Design review of the part built by this model. Coordinates are the model's own, in mm. A direction names the side the tool comes from. Coordinates: 2 decimals unless noted, no trailing zeros. Loops run counter-clockwise (first coordinate to the right, second up) from the corner with the lowest first, then second, coordinate; pieces in that order, holes last. Notation, with made-up numbers: (10.25, 12) -> (49.25, 12) arc R7 ccw to (49.25, 19) -> close; hole circle Ø10 at (45.25, 45). An arc over 180 degrees is marked (long way). Answer as a JSON object with one key per item and string values.
Autodesk Inventor part; units mm, degrees
ref_plane "YZ Plane" through (0, 0, 0) normal (1, 0, 0) x (0, 1, 0)
ref_plane "XZ Plane" through (0, 0, 0) normal (0, 1, 0) x (-1, 0, 0)
ref_plane "XY Plane" through (0, 0, 0) normal (0, 0, 1) x (1, 0, 0)
sketch "Sketch - Main Body" plane through (0, 0, 0) normal (0, 1, 0) x (-1, 0, 0)
  line L0 (-16.925, 11.65) -> (16.925, 11.65)
  line L1 (16.925, 11.65) -> (16.925, -11.65)
  line L2 (16.925, -11.65) -> (-16.925, -11.65)
  line L3 (-16.925, -11.65) -> (-16.925, 11.65)
  line L4 (-16.925, 11.65) -> (16.925, -11.65) construction
  line L5 (16.925, 11.65) -> (-16.925, -11.65) construction
  line L6 (-16.65, 11.25) -> (16.65, 11.25)
  line L7 (16.65, -11.25) -> (-16.65, -11.25)
  line L8 (-16.65, 11.25) -> (16.65, -11.25) construction
  line L9 (16.65, 11.25) -> (-16.65, -11.25) construction
  line L10 (16.65, 5) -> (12.65, 5)
  line L11 (12.65, 5) -> (12.65, -5)
  line L12 (12.65, -5) -> (16.65, -5)
  line L13 (-16.65, 5) -> (-12.65, 5)
  line L14 (-12.65, 5) -> (-12.65, -5)
  line L15 (-12.65, -5) -> (-16.65, -5)
  line L16 (16.65, 11.25) -> (16.65, 5)
  line L17 (16.65, -5) -> (16.65, -11.25)
  line L18 (-16.65, -11.25) -> (-16.65, -5)
  line L19 (-16.65, 5) -> (-16.65, 11.25)
  line L20 (-15.65, -10.25) -> (15.65, -10.25)
  line L21 (15.65, -10.25) -> (15.65, -6)
  line L22 (15.65, -6) -> (11.65, -6)
  line L23 (11.65, -6) -> (11.65, 6)
  line L24 (11.65, 6) -> (15.65, 6)
  line L25 (15.65, 6) -> (15.65, 10.25)
  line L26 (15.65, 10.25) -> (-15.65, 10.25)
  line L27 (-15.65, 10.25) -> (-15.65, 6)
  line L28 (-15.65, 6) -> (-11.65, 6)
  line L29 (-11.65, 6) -> (-11.65, -6)
  line L30 (-11.65, -6) -> (-15.65, -6)
  line L31 (-15.65, -6) -> (-15.65, -10.25)
  circle A0 centre (-14.1819, 8.9069) radius 2.7431
  circle A1 centre (14.1819, -8.9069) radius 2.7431
  point P0 (0, 0)
  point P1 (12.65, 0)
  point P2 (0, 0)
  dimension "d0" = 33.85
  dimension "d1" = 23.3
  dimension "d2" = 33.3
  dimension "d3" = 22.5
  dimension "d4" = 10
  dimension "d5" = 4
  dimension "d6" = 1
  dimension "d26" = 38.98
  dimension "d27" = 5.4863
extrude "Extrusion1" add sketch "Sketch - Main Body" against normal blind 1.35
extrude "Extrusion2" add sketch "Sketch - Main Body" along normal blind 8 contours A0 L26 L27 L19 L6 | L6 L16 L10 L11 L12 L17 A1 L21 L22 L23 L24 L25 L26 A0 | A0 L19 L6 | A0 L27 L28 L29 L30 L31 L20 A1 L7 L18 L15 L14 L13 L19 | L17 A1 L7 L20 L21 | L17 L7 A1
sketch "Sketch2" plane through (0, 0, 0) normal (0, 0, 1) x (1, 0, 0)
  line L0 (-11.65, 0) -> (-11.65, 21)
  line L1 (-15.65, 0) -> (-11.65, 0)
  line L2 (-11.65, 0) -> (-12.8159, 0)
  line L3 (-12.65, 0) -> (-16.65, 0)
  line L4 (-12.65, 0) -> (-12.65, 1.5)
  line L5 (-12.65, 0) -> (-12.65, 8)
  line L6 (-12.65, 1.5) -> (-13.65, 3.2321)
  line L7 (-13.65, 3.2321) -> (-13.65, 10.5)
  line L8 (-13.65, 10.5) -> (-14.55, 15)
  line L9 (-14.55, 15) -> (-14.8, 15)
  line L10 (-14.8, 15) -> (-14.8, 16.5)
  line L11 (-14.8, 16.5) -> (-12.65, 21)
  line L12 (-12.65, 21) -> (-11.65, 21)
  line L13 (-16.65, 0) -> (-16.65, 8)
  point P0 (0, 0)
  dimension "d11" = 1.5
  dimension "d12" = 1.5
  dimension "d13" = 3
  dimension "d14" = 30
  dimension "d15" = 3.15
  dimension "d16" = 1
  dimension "d17" = 4.5
  dimension "d18" = 21
  dimension "d19" = 10.5
  dimension "d20" = 0.25
extrude "Extrusion3" add sketch "Sketch2" along normal mid plane 12
mirror "Mirror1" about plane through (0, 0, 0) normal (1, 0, 0) of "Extrusion3"
fillet "Fillet1" radius 2.5 4 edges at (16.65, 4, 11.25) (16.65, 4, -11.25) (-16.65, 4, -11.25) (-16.65, 4, 11.25)
fillet "Fillet2" radius 2.75 4 edges at (16.925, -0.675, 11.65) (-16.925, -0.675, 11.65) (16.925, -0.675, -11.65) (-16.925, -0.675, -11.65)
properties part number "Toyota Yaris Aux Cap"
1) Clearance check with flat-ended pins moving along their axes: pin 1 Ø3 at (x, z) = (-4.5, 8) entering from +Y; pin 2 Ø1 at (y, z) = (5.5, -7.5) entering from -X; pin 3 Ø6 at (y, z) = (14, 4.5) entering from -X. State where each tip first meets the part, or that it passes through.
Completed:
{"pin 1": "y = 0", "pin 2": "x = -16.65", "pin 3": "x = -14.8"}
2) Wall thickness on probe 1 along Z at (x, y) = (-12, 6.5); probe 2 along Z at (x, y) = (10, 1); probe 3 along X at (y, z) = (6, -5.25): over which ranges is each line inside the solid? List them lowest first.
Completed:
{"probe 1": "-11.25 to -10.25, -6 to 6, 10.25 to 11.25", "probe 2": "-11.25 to -10.25, 10.25 to 11.25", "probe 3": "-16.65 to -11.65, 11.65 to 16.65"}
3) Add section D-D, the plane x = 11. Give the boundary of the cut face in (y, z), and give its area (3 significant figures).
Completed:
{"outline": "(-1.35, -11.65) -> (0, -11.65) -> (0, -11.25) -> (8, -11.25) -> (8, -10.25) -> (0, -10.25) -> (0, 10.25) -> (8, 10.25) -> (8, 11.25) -> (0, 11.25) -> (0, 11.65) -> (-1.35, 11.65) -> close", "area": "47.5 mm²"}
4) Add section A-A, the plane y = 12.5. Give the boundary of the cut face in (x, z).
Completed:
{"outline": "(-14.05, -6) -> (-11.65, -6) -> (-11.65, 6) -> (-14.05, 6) -> close; (11.65, -6) -> (14.05, -6) -> (14.05, 6) -> (11.65, 6) -> close"}
5) The part is to be moulded in two halves that separate along X. For faces 1 (the flat face through (-12, 21, 0)), 2 (the flat face through (-13.14, 2.35, -0.07)), 3 (the flat face through (-13, 8, 6)), say which applies: pulls with the +X half, pulls with the -X half, needs draft (parallel to the pull), parting line crosses it, or undercut.
Completed:
{"face 1": "needs draft", "face 2": "pulls with the -X half", "face 3": "undercut"}
6) Add section C-C, the plane y = 4.25. Give the boundary of the cut face in (x, z), and give its area (3 significant figures).
Completed:
{"outline": "(-16.65, -8.75) arc R2.5 ccw to (-14.15, -11.25) -> (14.15, -11.25) arc R2.5 ccw to (16.65, -8.75) -> (16.65, -5) -> (13.65, -5) -> (13.65, 5) -> (16.65, 5) -> (16.65, 8.75) arc R2.5 ccw to (14.15, 11.25) -> (-14.15, 11.25) arc R2.5 ccw to (-16.65, 8.75) -> (-16.65, 5) -> (-13.65, 5) -> (-13.65, -5) -> (-16.65, -5) -> close; hole (-15.65, -10.25) -> (15.65, -10.25) -> (15.65, -6) -> (11.65, -6) -> (11.65, 6) -> (15.65, 6) -> (15.65, 10.25) -> (-15.65, 10.25) -> (-15.65, 6) -> (-11.65, 6) -> (-11.65, -6) -> (-15.65, -6) -> close", "area": "138 mm²"}
7) Add section B-B, the plane z = 0.5. Give the boundary of the cut face in (x, y) (3 decimals), and give its area (3 significant figures).
Completed:
{"outline": "(-16.925, -1.35) -> (16.925, -1.35) -> (16.925, 0) -> (12.65, 0) -> (12.65, 1.5) -> (13.65, 3.232) -> (13.65, 10.5) -> (14.55, 15) -> (14.8, 15) -> (14.8, 16.5) -> (12.65, 21) -> (11.65, 21) -> (11.65, 0) -> (-11.65, 0) -> (-11.65, 21) -> (-12.65, 21) -> (-14.8, 16.5) -> (-14.8, 15) -> (-14.55, 15) -> (-13.65, 10.5) -> (-13.65, 3.232) -> (-12.65, 1.5) -> (-12.65, 0) -> (-16.925, 0) -> close", "area": "133 mm²"}
8) For faces 4 (the flat face through (-15, 4, -5)), 5 (the flat face through (-16.65, 4, 7)), 6 (the flat face through (-15.65, 4, 8)), 7 (the flat face through (16.65, 4, 7)), 8 (the flat face through (0, 4, -11.25)), list the 3-axis set-ups (+Z, -Z, +X, -X, +Y, -Y) from which the entire face can be reached by the end or side of a thin tool; tool diameter is ignored.
Completed:
{"face 4": "-X", "face 5": "+Z, -Z, -X, +Y", "face 6": "+Y", "face 7": "+Z, -Z, +X, +Y", "face 8": "-Z, +X, -X, +Y"}
